Autodesk Inventor part; units mm, degrees
ref_plane "Work Plane1" through (0, 0, 60.25) normal (0, 0, 1) x (1, 0, 0)
ref_plane "YZ Plane" through (0, 0, 0) normal (1, 0, 0) x (0, 1, 0)
ref_plane "XZ Plane" through (0, 0, 0) normal (0, 1, 0) x (-1, 0, 0)
sketch "Sketch2" plane through (0, 0, 0) normal (0, 1, 0) x (-1, 0, 0)
  line L0 (-45, 0) -> (7.5, 0)
  line L1 (0, -11.9711) -> (0, 71.8268)
  line L2 (-37.5, 0) -> (-37.5, 34)
  line L3 (-23.2693, 48.2307) -> (-23.6182, 59.8557)
  line L4 (-19.5, 55.9775) -> (-18, 6)
  line L5 (-19.5, 55.9775) -> (-23.6182, 59.8557)
  line L6 (-33.5, 0) -> (-37.5, 0)
  line L7 (-37.5, 34) -> (-23.2693, 48.2307)
  line L8 (-18, 6) -> (-24, 0)
  line L9 (-33.5, 0) -> (-24, 0)
  point P0 (0, 0)
  dimension "d4" = 4
  dimension "d7" = 34
  dimension "d8" = 37.5
  dimension "d9" = 18
  dimension "d10" = 50
  dimension "d11" = 135
  dimension "d15" = 19.5
  dimension "d25" = 24
  dimension "d26" = 45
  dimension "d27" = 135
revolve "Revolution1" add sketch "Sketch2" angle 360 about axis through (0, 0, -10) along (0, 0, 1)
fillet "Fillet1" radius 8 2 edges at (-23.2693, 0, 48.2307) (-37.5, 0, 34)
ref_plane "Work Plane1" through (0, 0, 60.25) normal (0, 0, 1) x (1, 0, 0)
sketch "Sketch3" plane through (0, 0, 60.25) normal (0, 0, 1) x (1, 0, 0)
  circle A0 centre (0, 0) radius 31.1812
extrude "Extrusion2" cut sketch "Sketch3" against normal blind 2
chamfer "Chamfer1" distance 0.5 angle 45 1 edges at (-37.5, 0, 0)
fillet "Fillet2" radius 8 1 edges at (-18, 0, 6)
properties part number "_3DPrint"
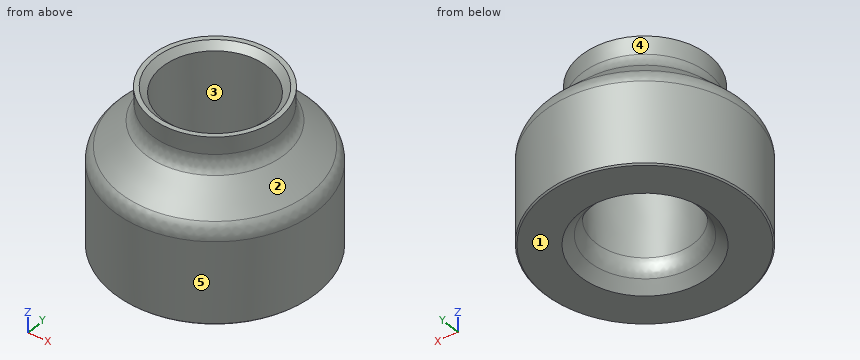
Design review of the part built by this model. Coordinates are the model's own, in mm. Face numbers are marked on the shaded views. A direction names the side the tool comes from. Coordinates: 2 decimals unless noted, no trailing zeros. Order: outer loops, then holes, each group sorted by start corner. A loop starts at its lowest first (then second) coordinate and runs counter-clockwise, first axis right, second up. Notation, with made-up numbers: (16.25, -1.5) -> (42.25, -1.5) arc R20 cw to (42.25, 28.5) -> close; hole circle Ø3 at (50, -29.5). An arc over 180 degrees is marked (long way). One line per item, written item: value.
1) To check wall thickness, follow probe 1 along X at (y, z) = (10, 8); probe 2 along Y at (x, z) = (-5.5, 33.5); probe 3 along X at (y, z) = (-7.5, 12). State the ranges of each line that lie inside material, in increasing order. Write a range as [from, to].
Output values:
probe 1: x = [-36.14, -15.2], [15.2, 36.14]
probe 2: y = [-36.58, -18], [18, 36.58]
probe 3: x = [-36.74, -16.56], [16.56, 36.74]
2) Clearance check with flat-ended pins moving along their axes: P1, Ø6, axis at x = 0, z = 18.5, coming from the +Y side; P2, Ø1, axis at y = 10.5, z = 36.5, coming from the +X side; P3, Ø1, axis at x = 27, z = 37.5, coming from the +Y side. State where each tip first meets the part, or that it passes through.
Output values:
P1: stops at y = 37.5
P2: stops at x = 33.92
P3: stops at y = 21.69
3) We need section A-A, the plane z = 17.5. Give the boundary of the cut face in (x, y).
Output values:
outline: circle Ø75 at (0, 0); hole circle Ø36.69 at (0, 0)
4) Draft analysis for pull direction Y (two halves, no side actions). For the marked faces 1, 2 and 3, state which applies: +Y half, -Y half, draft (parallel to the pull), parting line (faces both ways), or undercut.
Output values:
face 1: draft
face 2: parting line
face 3: undercut
5) Machinability: for the marked faces 4 and 5, which of the approach directions +Z, -Z, +X, -X, +Y, -Y give a long, thin tool a straight path to every point of the face, cutting with its end or side? Answer none if there is none.
Output values:
face 4: none
face 5: +Z, -Z
